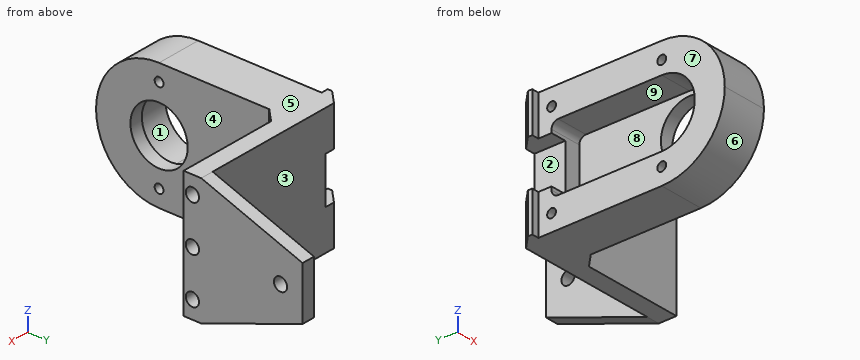
```python
from build123d import *

# Parameters (mm, degrees)
EXTRUDE_1_DEPTH          = 28.6
SKETCH_2_R               = 1
CUT_EXTRUDE_1_DEPTH      = 28.6
FILLET_1_R               = 14.3
CUT_EXTRUDE_2_DEPTH      = 7.3
CUT_EXTRUDE_4_DEPTH      = 19.6
CUT_EXTRUDE_4_DEPTH_BACK = 3.6
SKETCH_4_W               = 10.5
SKETCH_4_H               = 22.266748583
SKETCH_5_R               = 6.5
CUT_EXTRUDE_5_DEPTH      = 3.6
CUT_EXTRUDE_6_DEPTH      = 22.6
SKETCH_7_R               = 1.5
CUT_EXTRUDE_7_DEPTH      = 8


with BuildPart() as part:
    # Model → 凸台-拉伸1 (new body)
    with BuildSketch(Plane.XY):
        Polygon((-24.978787879, -17.92321671), (-14.678787879, -17.92321671), (-14.678787879, 21.376794113), (-11.678787879, 24.376794113), (11.321212121, 24.376794113), (11.321212121, 51.376794114), (8.321212121, 51.376794114), (8.321212121, 28.376794114), (-23.578787879, 28.376794114), (-26.578787879, 25.376794114), (-26.578787879, 24.376794113), (-24.978787879, 24.376794113), align=None)
    extrude(amount=EXTRUDE_1_DEPTH)

    # 草图2 → 切除-拉伸1 (cut)
    with BuildSketch(Plane.ZY.offset(24.978787879)):
        with Locations((3.78, 21.376794113)):
            Circle(SKETCH_2_R)
        with Locations((24.78, 21.376794113)):
            Circle(SKETCH_2_R)
        with Locations((24.82, -3.623205887)):
            Circle(SKETCH_2_R)
        with Locations((3.82, -3.623205887)):
            Circle(SKETCH_2_R)
    extrude(amount=-CUT_EXTRUDE_1_DEPTH, mode=Mode.SUBTRACT)

    # 圆角1
    fillet_1_edges = [part.edges().sort_by_distance(p)[0] for p in [
        (-19.828787879, -17.92321671, 28.6),
        (-19.828787879, -17.92321671, 0),
    ]]
    fillet(fillet_1_edges, radius=FILLET_1_R - 0.0001)  # a hair under: the kernel refuses the full size

    # 草图3 → 切除-拉伸2 (cut)
    with BuildSketch(Plane.ZY.offset(24.978787879)):
        with BuildLine():
            Line((21.8, -3.62321671), (21.8, 19.87678329))
            ThreePointArc((21.8, 19.87678329), (21.360660172, 20.937443461), (20.3, 21.37678329))
            Line((20.3, 21.37678329), (8.3, 21.37678329))
            ThreePointArc((8.3, 21.37678329), (7.239339828, 20.937443461), (6.8, 19.87678329))
            Line((6.8, 19.87678329), (6.8, -3.62321671))
            ThreePointArc((6.8, -3.62321671), (14.3, -11.12321671), (21.8, -3.62321671))
        make_face()
    extrude(amount=-CUT_EXTRUDE_2_DEPTH, mode=Mode.SUBTRACT)

    # 草图4 → 切除-拉伸4 (cut, two sides: drawn at the far end of the back side and taken through both)
    with BuildSketch(Plane.ZY.offset(24.978787879).offset(-CUT_EXTRUDE_4_DEPTH_BACK)):
        with Locations((14.3, 25.815793082)):
            Rectangle(SKETCH_4_W, SKETCH_4_H)
    extrude(amount=CUT_EXTRUDE_4_DEPTH + CUT_EXTRUDE_4_DEPTH_BACK, mode=Mode.SUBTRACT)

    # 草图5 → 切除-拉伸5 (cut)
    with BuildSketch(Plane.ZY.offset(17.678787879)):
        with Locations((14.3, -3.62321671)):
            Circle(SKETCH_5_R)
    extrude(amount=-CUT_EXTRUDE_5_DEPTH, mode=Mode.SUBTRACT)

    # 草图6 → 切除-拉伸6 (cut)
    with BuildSketch(Plane(origin=(11.321212121, 0, 0), x_dir=(0, 0, -1), z_dir=(1, 0, 0))):
        Polygon((0, 28.376794114), (-8.3, 51.376794114), (5.727876299, 54.90154804), align=None)
        Polygon((-20.3, 51.376794114), (-28.6, 28.376794114), (-35.26481715, 54.90154804), align=None)
    extrude(amount=-CUT_EXTRUDE_6_DEPTH, mode=Mode.SUBTRACT)

    # 草图7 → 切除-拉伸7 (cut)
    with BuildSketch(Plane(origin=(11.321212121, 0, 0), x_dir=(0, 0, -1), z_dir=(1, 0, 0))):
        with Locations((-14.3, 46.376794114)):
            Circle(SKETCH_7_R)
        with Locations((-24.6, 26.376794113)):
            Circle(SKETCH_7_R)
        with Locations((-14.3, 26.376794113)):
            Circle(SKETCH_7_R)
        with Locations((-4, 26.376794113)):
            Circle(SKETCH_7_R)
    extrude(amount=-CUT_EXTRUDE_7_DEPTH, mode=Mode.SUBTRACT)


solid = part.part
```
Part model, mm, in its own coordinate system. Face numbers are marked on the shaded views. A direction names the side the tool comes from. Coordinates: 2 decimals unless noted, no trailing zeros. Order: outer loops, then holes, each group sorted by start corner. A loop starts at its lowest first (then second) coordinate and runs counter-clockwise, first axis right, second up. Notation, with made-up numbers: (89, 20) -> (117, 20) arc R26 cw to (117, 44) -> close; hole circle Ø6 at (11.5, 72). An arc over 180 degrees is marked (long way). Put each result on its own line as item: value. Start each with the question number.
(1) Which spindle directions (+Z, -Z, +X, -X, +Y, -Y) get a long thin tool onto all of the face, cutting with end or side? Do the marked faces 1, 2, 3, 4 and 5. Say none if no direction does.
(2) Probe line 1 along Z through (x, y) = (-20, 10.5); line 2 along Y through (x, z) = (-18, 3.78); line 3 along Y through (x, z) = (-22.5, 25). List the from-to ranges inside material, lowest first. Write a range as [from, to].
(3) Band-saw the part on A-A (y = -8). Give the cut face in (x, z), then the cut area to 3 significant figures.
(4) Band-saw the part on C-C (x = -5.5). Give the cut face in (y, z), then the cut area to 3 significant figures.
(5) Pin check, flat tips, straight feed: pin 1 Ø0.9 at (y, z) = (26, 3.5) entering from +X; pin 2 Ø1.6 at (y, z) = (-3.62, 24.82) entering from +X; pin 3 Ø5 at (y, z) = (7, 4.5) entering from +X; pin 4 Ø1.8 at (x, z) = (-25.5, 6.5) entering from -Y. Stop position of each tip, or through.
(6) Mould opens along Y. For the marked faces 6, 7, 8 and 9 say: pulls with the +Y half, pulls with the -Y half, needs draft (parallel to the pull), parting line crosses it, or undercut.
(7) Band-saw the part on D-D (z = 4). Give the cut face in (x, y).
(8) Band-saw the part on B-B (z = 24.78). Give the cut face in (x, y), then the cut area to 3 significant figures.
Determined:
1. face 1: -X
1. face 2: -X, +Y
1. face 3: +Z, -Z, -X, +Y
1. face 4: +Z, -Z, +X, -Y
1. face 5: +Z, +X, -X, +Y, -Y
2. line 1: z = [0, 6.8], [21.8, 28.6]
2. line 2: y = [-13.31, -4.62], [-2.62, 20.38], [22.38, 28.38]
2. line 3: y = [-13.11, -4.61], [-2.64, 20.4], [22.35, 28.38]
3. outline: (-24.98, 0.69) -> (-14.68, 0.69) -> (-14.68, 9.49) -> (-17.68, 9.49) -> (-17.68, 8.21) -> (-24.98, 8.21) -> close; (-24.98, 20.39) -> (-17.68, 20.39) -> (-17.68, 19.11) -> (-14.68, 19.11) -> (-14.68, 27.91) -> (-24.98, 27.91) -> close
3. area: 163 mm²
4. outline: (24.38, 0) -> (28.38, 0) -> (28.38, 28.6) -> (24.38, 28.6) -> close
4. area: 114 mm²
5. pin 1: stops at x = 3.32
5. pin 2: passes through
5. pin 3: stops at x = -14.68
5. pin 4: stops at y = -16.06
6. face 6: pulls with the -Y half
6. face 7: needs draft
6. face 8: undercut
6. face 9: undercut
7. outline: (-26.58, 24.38) -> (-24.98, 24.38) -> (-24.98, 22.35) -> (-13.7, 22.35) -> (-11.68, 24.38) -> (11.32, 24.38) -> (11.32, 24.88) -> (3.32, 24.88) -> (3.32, 27.88) -> (11.32, 27.88) -> (11.32, 39.46) -> (8.32, 39.46) -> (8.32, 28.38) -> (-23.58, 28.38) -> (-26.58, 25.38) -> close; (-24.98, -13.54) -> (-14.68, -13.54) -> (-14.68, -4.61) -> (-24.98, -4.61) -> close; (-24.98, -2.64) -> (-14.68, -2.64) -> (-14.68, 20.4) -> (-24.98, 20.4) -> close
8. outline: (-26.58, 24.38) -> (-24.98, 24.38) -> (-24.98, 22.38) -> (-13.68, 22.38) -> (-11.68, 24.38) -> (11.32, 24.38) -> (11.32, 24.89) -> (3.32, 24.89) -> (3.32, 27.87) -> (11.32, 27.87) -> (11.32, 38.96) -> (8.32, 38.96) -> (8.32, 28.38) -> (-23.58, 28.38) -> (-26.58, 25.38) -> close; (-24.98, -13.35) -> (-14.68, -13.35) -> (-14.68, -4.62) -> (-24.98, -4.62) -> close; (-24.98, -2.62) -> (-14.68, -2.62) -> (-14.68, 20.38) -> (-24.98, 20.38) -> close
8. area: 506 mm²
